Geometry: final body of the model. Coordinates: model frame, mm. A direction names the side the tool comes from. Give positions to 0.01 mm unless a question says otherwise; leave off trailing zeros. Order: outer loops, then holes, each group sorted by start corner. A loop starts at its lowest first (then second) coordinate and runs counter-clockwise, first axis right, second up. Notation, with made-up numbers: (17.5, 49) - (40.5, 49) arc R25 cw to (40.5, 88) - close; hole circle Ø7 at (-19, -27). An arc over 180 degrees is marked (long way). Write item = value, one per line. Start each with the question number.
from build123d import *

# Parameters (mm, degrees)
BOSS_EXTRUDE1_DEPTH = 7.82
SKETCH2_R           = 2.445
BOSS_EXTRUDE2_DEPTH = 1.93
SKETCH3_R           = 2.375
SKETCH3_R_2         = 1.595
BOSS_EXTRUDE3_DEPTH = 1.67
SHELL1_START        = -3.16
SHELL1_OUTLINE_W    = 6.43
SHELL1_OUTLINE_H    = 4.62
SHELL1_DEPTH        = 1.56
SHELL1_START_2      = -1.6
SHELL1_2_OUTLINE_R  = 0.845
SHELL1_2_DEPTH      = 1.93
FILLET1_R           = 1


# Read off the part's stored shape, not the designer's step: Shell1
with BuildPart() as part:
    # Sketch1 → Boss-Extrude1 (new body)
    with BuildSketch(Plane.XY):
        Polygon((0, 0), (-8.02, 0), (-8.02, -3.16), (1.61, -3.16), (1.61, 4.81), (0, 4.81), align=None)
    extrude(amount=-BOSS_EXTRUDE1_DEPTH)

    # Sketch2 → Boss-Extrude2 (add)
    with BuildSketch(Plane(origin=(0, 0, 0), x_dir=(1, 0, 0), z_dir=(0, 1, 0))):
        with Locations(Location((-4.01, 3.91, 0), (0, 0, 180))):
            Circle(SKETCH2_R)
    extrude(amount=BOSS_EXTRUDE2_DEPTH)

    # Sketch3 → Boss-Extrude3 (add)
    with BuildSketch(Plane(origin=(1.61, 0, 0), x_dir=(0, 0, -1), z_dir=(1, 0, 0))):
        with Locations(Location((3.91, 0.825, 0), (0, 0, 90))):
            Circle(SKETCH3_R)
        with Locations(Location((3.91, 0.825, 0), (0, 0, 90))):
            Circle(SKETCH3_R_2, mode=Mode.SUBTRACT)
    extrude(amount=BOSS_EXTRUDE3_DEPTH)

    # Shell1 outline → Shell1 (cut)
    with BuildSketch(Plane(origin=(0, 0, 0), x_dir=(1, 0, 0), z_dir=(0, 1, 0)).offset(SHELL1_START)):
        with Locations((-3.205, 3.91)):
            Rectangle(SHELL1_OUTLINE_W, SHELL1_OUTLINE_H)
    extrude(amount=SHELL1_DEPTH, mode=Mode.SUBTRACT)

    # Shell1 2 outline → Shell1 2 (cut)
    with BuildSketch(Plane(origin=(0, 0, 0), x_dir=(1, 0, 0), z_dir=(0, 1, 0)).offset(SHELL1_START_2)):
        with Locations((-4.01, 3.91)):
            Circle(SHELL1_2_OUTLINE_R)
    extrude(amount=SHELL1_2_DEPTH, mode=Mode.SUBTRACT)

    # Fillet1
    fillet1_edges = [part.edges().sort_by_distance(p)[0] for p in [
        (0.805, 4.81, -7.82),
        (0.805, 4.81, 0),
    ]]
    fillet(fillet1_edges, radius=FILLET1_R)


solid = part.part
Q1. Material intervals for line 1 along X through (y, z) = (-0.2, -3.91) (3 decimals); line 2 along X through (y, z) = (-2, -5); line 3 along Z through (x, y) = (-4.5, -2.5), sorted ascending. Write a range as from..to.
Q2. Section D-D, the plane z = -3.91. Return the cut outline in (x, y) (3 decimals).
Q3. Contact query for flat-ended pins moving along their axis: pin 1 (1.2 mm diameter, centred on y = -2.5, z = -5, fed in from +X); pin 2 (1 mm diameter, centred on x = -4, y = 3, fed in from +Z); pin 3 (0.5 mm diameter, centred on x = -4.5, z = -3.5, fed in from -Y); pin 4 (2.5 mm diameter, centred on x = -3.5, z = -4.5, fed in from +Y). Output: stop coordinate, or through.
Q4. Section B-B, the plane x = -4.01. Return the cut outline in (y, z) (3 decimals).
Q5. Set-up query: faces 1 (the flat face through (0, 2, -4)), 2 (the flat face through (1.61, 3, -2)), 3 (the cylindrical face through (-3.5, 1, -6.3)), 4 (the flat face through (-3, -1, -7.82)), 5 (the flat face through (-3, -2, -6.22)). Return all of +Z, -Z, +X, -X, +Y, -Y with unobstructed straight access to the full face (end or side cutting, diameter ignored); none if empty.
Q6. Pull-direction query (Z, two-part tool) for faces 6 (the flat face through (-3, -1, 0)), 7 (the flat face through (1.61, 1, -4)), 8 (the cylindrical face through (2.43, 0.31, -6.23)); classes: +Z half, -Z half, draft (parallel to the pull), parting line (faces both ways), or undercut.
Q7. Section C-C, the plane y = -0.5. Return the cut outline in (x, z) (3 decimals), then the cut area to 3 significant figures.
Q8. Section A-A, the plane y = 1.5. Return the cut outline in (x, z) (3 decimals), then the cut area to 3 significant figures.
The answers:
q1.line_1 = -8.02..-4.855, -3.165..1.61
q1.line_2 = -8.02..-6.42, 0.01..1.61
q1.line_3 = -7.82..-6.22, -1.6..0
q2.outline = (-8.02, -3.16) - (-6.42, -3.16) - (-6.42, -1.6) - (-4.855, -1.6) - (-4.855, 0.33) - (-3.165, 0.33) - (-3.165, -1.6) - (0.01, -1.6) - (0.01, -3.16) - (1.61, -3.16) - (1.61, -1.55) - (3.28, -1.55) - (3.28, -0.77) - (1.61, -0.77) - (1.61, 2.42) - (3.28, 2.42) - (3.28, 3.2) - (1.61, 3.2) - (1.61, 4.81) - (0, 4.81) - (0, 0) - (-1.565, 0) - (-1.565, 1.93) - (-6.455, 1.93) - (-6.455, 0) - (-8.02, 0) - close
q3.pin_1 = 1.61
q3.pin_2 = through
q3.pin_3 = -1.6
q3.pin_4 = 1.93
q4.outline = (-3.16, -7.82) - (0, -7.82) - (0, -6.355) - (1.93, -6.355) - (1.93, -1.465) - (0, -1.465) - (0, 0) - (-3.16, 0) - (-3.16, -1.6) - (-1.6, -1.6) - (-1.6, -3.065) - (0.33, -3.065) - (0.33, -4.755) - (-1.6, -4.755) - (-1.6, -6.22) - (-3.16, -6.22) - close
q5.face_1 = +Z, -Z, +Y
q5.face_2 = +X
q5.face_3 = +Y
q5.face_4 = -Z, +X, -X, +Y, -Y
q5.face_5 = -Y
q6.face_6 = +Z half
q6.face_7 = undercut
q6.face_8 = parting line
q7.outline = (-8.02, -7.82) - (1.61, -7.82) - (1.61, -5.881) - (3.28, -5.881) - (3.28, -4.798) - (1.61, -4.798) - (1.61, -3.022) - (3.28, -3.022) - (3.28, -1.939) - (1.61, -1.939) - (1.61, 0) - (-8.02, 0) - close; hole circle Ø1.69 at (-4.01, -3.91)
q7.area = 76.7 mm²
q8.outline = circle Ø4.89 at (-4.01, -3.91); (0, -7.82) - (1.61, -7.82) - (1.61, -6.187) - (3.28, -6.187) - (3.28, -5.355) - (1.61, -5.355) - (1.61, -2.465) - (3.28, -2.465) - (3.28, -1.633) - (1.61, -1.633) - (1.61, 0) - (0, 0) - close
q8.area = 34.1 mm²
